The model under review builds one solid part; all positions refer to its coordinate system, in mm. Round coordinates to 2 decimals unless told otherwise and drop trailing zeros. Write each loop counter-clockwise with the first axis right and the second up, starting at its lowest first coordinate (ties: lowest second). Pieces come first, ordered by that corner, then holes. Notation, with made-up numbers: M -4,16.5 L 43,16.5 A25 cw 43,31.5 Z; hole C 27,5 d5. An arc over 180 degrees is marked long. Write item = value, one per line. Start each with the question number.
Item 1: To check wall thickness, follow line 1 along Y through (x, z) = (-27.94, -17.6). State the ranges of the line that lie inside material, in increasing order.
Item 2: The part is to be moulded in two halves that separate along Y. For faces 1 (the cylindrical face through (-28.448, 28.916, -17.866)), 2 (the flat face through (0, 0, -17.25)), say which applies: +Y half, -Y half, draft (parallel to the pull), parting line (faces both ways), or undercut.
Item 3: Take a section at A-A, the plane y = -27.94. Give the boundary of the cut face in (x, z).
Autodesk Inventor part; units mm, degrees
ref_plane "YZ Plane" through (0, 0, 0) normal (1, 0, 0) x (0, 1, 0)
ref_plane "XZ Plane" through (0, 0, 0) normal (0, 1, 0) x (-1, 0, 0)
ref_plane "XY Plane" through (0, 0, 0) normal (0, 0, 1) x (1, 0, 0)
sketch "Skizze1" plane through (0, 0, 0) normal (0, 0, 1) x (1, 0, 0)
  line L0 (-33.02, -33.02) -> (33.02, -33.02)
  line L1 (33.02, -33.02) -> (33.02, 33.02)
  line L2 (33.02, 33.02) -> (-33.02, 33.02)
  line L3 (-33.02, 33.02) -> (-33.02, -33.02)
  line L4 (-33.02, -33.02) -> (33.02, 33.02) construction
  line L5 (33.02, -33.02) -> (-33.02, 33.02) construction
  line L6 (-34, -34) -> (34, -34)
  line L7 (34, -34) -> (34, 34)
  line L8 (34, 34) -> (-34, 34)
  line L9 (-34, 34) -> (-34, -34)
  line L10 (-34, -34) -> (34, 34) construction
  line L11 (34, -34) -> (-34, 34) construction
  point P0 (0, 0)
  dimension "d0" = 66.04
  dimension "d1" = 66.04
  dimension "d2" = 68
  dimension "d3" = 68
extrude "Extrusion1" add sketch "Skizze1" along normal blind 6.5
sketch "Skizze2" plane through (0, 0, 6.5) normal (0, 0, 1) x (1, 0, 0)
  line L0 (-33.02, 33.02) -> (33.02, 33.02)
  line L1 (-33.02, -33.02) -> (33.02, -33.02)
  line L2 (33.02, -33.02) -> (33.02, 33.02)
  line L3 (33.02, 33.02) -> (-33.02, 33.02)
  line L4 (-33.02, 33.02) -> (-33.02, -33.02)
  line L5 (-33.02, -33.02) -> (33.02, 33.02) construction
  line L6 (33.02, -33.02) -> (-33.02, 33.02) construction
  line L7 (34, -34) -> (34, 34)
  line L8 (34, 34) -> (-34, 34)
  line L9 (-34, 34) -> (-34, -34)
  line L10 (-34, -34) -> (34, -34)
  line L11 (-33.02, -33.02) -> (-33.02, 33.02)
  line L12 (-33.02, 33.02) -> (33.02, 33.02)
  line L13 (33.02, 33.02) -> (33.02, -33.02)
  line L14 (33.02, -33.02) -> (-33.02, -33.02)
  point P0 (0, 0)
extrude "Extrusion2" add sketch "Skizze2" along normal blind 2 contours L0 L2 L1 L4 | L10 L9 L8 L7
sketch "Skizze3" plane through (0, 0, 6.5) normal (0, 0, -1) x (-1, 0, 0)
  line L0 (-27.94, -27.94) -> (27.94, -27.94)
  line L1 (27.94, -27.94) -> (27.94, 27.94)
  line L2 (27.94, 27.94) -> (-27.94, 27.94)
  line L3 (-27.94, 27.94) -> (-27.94, -27.94)
  line L4 (-27.94, -27.94) -> (27.94, 27.94) construction
  line L5 (27.94, -27.94) -> (-27.94, 27.94) construction
  circle A0 centre (-27.94, 27.94) radius 3.35
  circle A1 centre (27.94, 27.94) radius 3.35
  circle A2 centre (27.94, -27.94) radius 3.35
  circle A3 centre (-27.94, -27.94) radius 3.35
  point P0 (0, 0)
  dimension "d8" = 55.88
  dimension "d9" = 55.88
  dimension "d10" = 6.7
  dimension "d11" = 6.7
  dimension "d12" = 6.7
  dimension "d13" = 6.7
extrude "Extrusion3" add sketch "Skizze3" along normal blind 5 contours L3 A3 L0 | L0 A3 L3 | A2 L1 L0 | L0 L1 A2 | A0 L2 L3 | L3 L2 A0 | A1 L2 L1 | L1 L2 A1
sketch "Skizze4" plane through (27.94, 27.94, 1.5) normal (0, 0, -1) x (-1, 0, 0)
  circle A0 centre (0, 0) radius 1.1
  circle A1 centre (55.88, 0) radius 3.35
  circle A2 centre (55.88, 0) radius 1.1
  circle A3 centre (55.88, -55.88) radius 3.35
  circle A4 centre (55.88, -55.88) radius 1.1
  circle A5 centre (0, -55.88) radius 3.35
  circle A6 centre (0, -55.88) radius 1.1
  point P0 (27.94, -27.94)
  dimension "d17" = 2.2
  dimension "d18" = 2.2
  dimension "d19" = 2.2
  dimension "d20" = 2.2
extrude "Extrusion4" cut sketch "Skizze4" against normal blind 5 contours A0 | A2 | A4 | A6
sketch "Skizze5" plane through (0, 0, 0) normal (0, 0, -1) x (-1, 0, 0)
  line L0 (-34, -34) -> (-34, 34)
  line L1 (34, -34) -> (-34, -34)
  line L2 (34, 34) -> (34, -34)
  line L3 (-34, 34) -> (34, 34)
  line L4 (33.02, -33.02) -> (33.02, 33.02)
  line L5 (-33.02, -33.02) -> (33.02, -33.02)
  line L6 (-33.02, 33.02) -> (-33.02, -33.02)
  line L7 (33.02, 33.02) -> (-33.02, 33.02)
  point P0 (0, 0)
extrude "Extrusion5" add sketch "Skizze5" along normal blind 4
sketch "Skizze6" plane through (0, 0, -4) normal (0, 0, -1) x (-1, 0, 0)
  line L0 (-33.02, -33.02) -> (33.02, -33.02)
  line L1 (33.02, -33.02) -> (33.02, 33.02)
  line L2 (33.02, 33.02) -> (-33.02, 33.02)
  line L3 (-33.02, 33.02) -> (-33.02, -33.02)
  line L4 (-33.02, -33.02) -> (33.02, 33.02) construction
  line L5 (33.02, -33.02) -> (-33.02, 33.02) construction
  line L6 (33.02, -33.02) -> (20.02, -33.02)
  line L7 (-33.02, -33.02) -> (33.02, -33.02)
  line L8 (20.02, -33.02) -> (10.08, -33.02)
  line L9 (34, -34) -> (-34, -34)
  line L10 (10.08, -33.02) -> (20.02, -33.02)
  line L11 (20.02, -33.02) -> (20.02, -34)
  line L12 (20.02, -34) -> (10.08, -34)
  line L13 (10.08, -34) -> (10.08, -33.02)
  point P0 (0, 0)
  point P1 (-24.13, -33.02)
  point P2 (24.13, -33.02)
  dimension "d25" = 66.04
  dimension "d26" = 66.04
  dimension "d27" = 13
  dimension "d28" = 9.94
extrude "Extrusion6" cut sketch "Skizze6" against normal blind 4 contours L0 L11 L9 L13
fillet "Rundung2" radius 1.75 2 edges at (-10.08, -33.51, 0) (-20.02, -33.51, 0)
sketch "Skizze7" plane through (0, 0, -4) normal (0, 0, -1) x (-1, 0, 0)
  line L0 (34, 34) -> (-34, 34)
  line L1 (-34, -34) -> (34, -34)
  line L2 (34, -34) -> (34, 34)
  line L3 (34, 34) -> (-34, 34)
  line L4 (-34, 34) -> (-34, -34)
  line L5 (-34, -34) -> (34, 34) construction
  line L6 (34, -34) -> (-34, 34) construction
  line L7 (-35, -35) -> (35, -35)
  line L8 (35, -35) -> (35, 35)
  line L9 (35, 35) -> (-35, 35)
  line L10 (-35, 35) -> (-35, -35)
  line L11 (-35, -35) -> (35, 35) construction
  line L12 (35, -35) -> (-35, 35) construction
  point P0 (0, 0)
  point P1 (-34, 34)
  dimension "d32" = 70
  dimension "d33" = 70
extrude "Extrusion7" add sketch "Skizze7" against normal up to surface (12.5 mm away)
sketch "Skizze8" plane through (-20.02, -34, -4) normal (0, 1, 0) x (1, 0, 0)
  line L0 (9.94, -2.25) -> (9.94, 0)
  line L1 (0, 0) -> (9.94, 0)
  line L2 (0, 0) -> (0, -2.25)
  arc A0 (0, -2.25) -> (1.75, -4) centre (1.75, -2.25) ccw
  line L3 (1.75, -4) -> (8.19, -4)
  arc A1 (8.19, -4) -> (9.94, -2.25) centre (8.19, -2.25) ccw
  point P0 (20.02, -4)
extrude "Extrusion8" cut sketch "Skizze8" against normal blind 10
sketch "Skizze9" plane through (0, 0, -4) normal (0, 0, -1) x (-1, 0, 0)
  line L0 (-33.52, 33.52) -> (33.52, 33.52)
  line L1 (33.52, 33.52) -> (33.52, -33.52)
  line L2 (33.52, -33.52) -> (-33.52, -33.52)
  line L3 (-33.52, -33.52) -> (-33.52, 33.52)
  line L4 (-33.52, 33.52) -> (33.52, -33.52) construction
  line L5 (33.52, 33.52) -> (-33.52, -33.52) construction
  line L6 (10.08, -35) -> (10.08, -33.02)
  line L7 (10.08, -33.02) -> (-33.02, -33.02)
  line L8 (-33.02, -33.02) -> (-33.02, 33.02)
  line L9 (-33.02, 33.02) -> (33.02, 33.02)
  line L10 (33.02, 33.02) -> (33.02, -33.02)
  line L11 (33.02, -33.02) -> (20.02, -33.02)
  line L12 (20.02, -33.02) -> (20.02, -35)
  line L13 (20.02, -35) -> (35, -35)
  line L14 (35, -35) -> (35, 35)
  line L15 (35, 35) -> (-35, 35)
  line L16 (-35, 35) -> (-35, -35)
  line L17 (-35, -35) -> (10.08, -35)
  point P0 (0, 0)
  point P1 (10.08, -33.52)
  point P2 (20.02, -33.52)
  dimension "d38" = 67.04
  dimension "d39" = 67.04
extrude "Extrusion9" cut sketch "Skizze9" against normal up to surface (10.5 mm away) contours L0 L1 L2 L12 L11 L10 L9 L8 L7 L6 L3
fillet "Rundung3" radius 2 4 edges at (31.29, -27.94, 6.5) (31.29, 27.94, 6.5) (-24.59, 27.94, 6.5) (-24.59, -27.94, 6.5)
sketch "Skizze10" plane through (-35, -35, -4) normal (-1, 0, 0) x (0, 0, 1)
  point P0 (4, 35)
sketch "Skizze11" plane through (0, 0, 8.5) normal (0, 0, 1) x (1, 0, 0)
  point P0 (0, 0)
sketch "Skizze12" plane through (-18.27, -33.02, 0) normal (0, 1, 0) x (1, 0, 0)
  line L0 (-1.75, 1.75) -> (-1.75, -6.5)
  line L1 (8.19, -6.5) -> (-1.75, -6.5)
  line L2 (8.19, -6.5) -> (8.19, 1.75)
  arc A0 (6.44, 0) -> (8.19, 1.75) centre (6.44, 1.75) ccw
  line L3 (6.44, 0) -> (0, 0)
  arc A1 (-1.75, 1.75) -> (0, 0) centre (0, 1.75) ccw
  point P0 (18.27, 0)
extrude "Extrusion10" cut sketch "Skizze12" against normal up to surface (0.5 mm away)
sketch "Skizze13" plane through (0, 0, -4) normal (0, 0, -1) x (-1, 0, 0)
  circle A0 centre (0, 0) radius 4
  line L0 (0, 0) -> (-10.0581, 1.7135)
  line L1 (0, 0) -> (10.203, 0) construction
  line L2 (0, 0) -> (1.8539, 9.7483)
  line L3 (0, 0) -> (9.923, 0) construction
  line L4 (0, 0) -> (9.888, -2.1637)
  line L5 (0, 0) -> (10.122, 0) construction
  line L6 (0, 0) -> (-2.0234, -10.1982)
  line L7 (0, 0) -> (10.397, 0) construction
  circle A1 centre (-2.0234, -10.1982) radius 2.5
  circle A2 centre (-10.0581, 1.7135) radius 2.5
  circle A3 centre (1.8539, 9.7483) radius 2.5
  circle A4 centre (9.888, -2.1637) radius 2.5
  dimension "d59" = 8
  dimension "d60" = 10.203
  dimension "d61" = 170.332
  dimension "d62" = 9.923
  dimension "d63" = 79.232
  dimension "d64" = 10.122
  dimension "d65" = 12.343
  dimension "d66" = 10.397
  dimension "d67" = 101.222
  dimension "d68" = 5
  dimension "d69" = 5
  dimension "d70" = 5
  dimension "d71" = 5
extrude "Extrusion11" add sketch "Skizze13" against normal up to surface (10.5 mm away) contours A1 | A2 | A3 | A4
sketch "Skizze14" plane through (-9.888, -2.1637, -4) normal (0, 0, -1) x (-1, 0, 0)
  circle A0 centre (0, 0) radius 2.5
  circle A1 centre (-11.9114, -8.0345) radius 2.5
  circle A2 centre (-19.9461, 3.8772) radius 2.5
  circle A3 centre (-8.0341, 11.912) radius 2.5
  point P0 (-9.888, 2.1637)
extrude "Extrusion12" cut sketch "Skizze14" against normal blind 5.5
fillet "Rundung4" radius 4 4 edges at (12.5581, 1.7135, 6.5) (0.6461, 9.7483, 6.5) (-7.388, -2.1637, 6.5) (4.5234, -10.1982, 6.5)
sketch "Skizze15" plane through (-9.888, -2.1637, 1.5) normal (0, 0, -1) x (-1, 0, 0)
  circle A0 centre (0, 0) radius 1
  circle A1 centre (-11.9114, -8.0345) radius 2.5
  circle A2 centre (-11.9114, -8.0345) radius 1
  circle A3 centre (-19.9461, 3.8772) radius 2.5
  circle A4 centre (-19.9461, 3.8772) radius 1
  circle A5 centre (-8.0341, 11.912) radius 2.5
  circle A6 centre (-8.0341, 11.912) radius 1
  point P0 (-9.888, 2.1637)
  dimension "d77" = 2
  dimension "d78" = 2
  dimension "d79" = 2
  dimension "d80" = 2
extrude "Extrusion13" cut sketch "Skizze15" against normal blind 5 contours A0 | A2 | A4 | A6
chamfer "Fase1" distance 4 angle 45 4 edges at (-33.52, 0, 6.5) (0, -33.52, 6.5) (0, 33.52, 6.5) (33.52, 0, 6.5)
sketch "Skizze16" plane through (10.0581, 1.7135, 1.5) normal (0, 0, -1) x (-1, 0, 0)
  circle A0 centre (0, 0) radius 1.6
  circle A1 centre (8.0347, -11.9117) radius 1
  circle A2 centre (8.0347, -11.9117) radius 1.6
  circle A3 centre (11.912, 8.0348) radius 1
  circle A4 centre (11.912, 8.0348) radius 1.6
  circle A5 centre (19.9461, -3.8772) radius 1
  circle A6 centre (19.9461, -3.8772) radius 1.6
  point P0 (10.0581, -1.7135)
  dimension "d86" = 3.2
  dimension "d87" = 3.2
  dimension "d88" = 3.2
  dimension "d89" = 3.2
extrude "Extrusion14" cut sketch "Skizze16" against normal blind 10 contours A0 | A1 | A2 | A3 | A4 | A5 | A6
chamfer "Fase2" distance 2 angle 45 4 edges at (-8.288, -2.1637, 8.5) (3.6234, -10.1982, 8.5) (11.6581, 1.7135, 8.5) (-0.2539, 9.7483, 8.5)
sketch "Skizze17" plane through (27.94, 27.94, 1.5) normal (0, 0, -1) x (-1, 0, 0)
  circle A0 centre (0, 0) radius 1.1
  circle A1 centre (0, 0) radius 3.35
  circle A2 centre (55.88, 0) radius 1.1
  circle A3 centre (55.88, 0) radius 3.35
  circle A4 centre (55.88, -55.88) radius 1.1
  circle A5 centre (55.88, -55.88) radius 3.35
  circle A6 centre (0, -55.88) radius 1.1
  circle A7 centre (0, -55.88) radius 3.35
  line L0 (61.46, 5.58) -> (58.4446, 2.5646)
  line L1 (-2.5646, -58.4446) -> (58.4446, -58.4446)
  line L2 (58.4446, -58.4446) -> (58.4446, 2.5646)
  line L3 (58.4446, 2.5646) -> (-2.5646, 2.5646)
  line L4 (-2.5646, 2.5646) -> (-2.5646, -58.4446)
  line L5 (-2.5646, -58.4446) -> (58.4446, 2.5646) construction
  line L6 (58.4446, -58.4446) -> (-2.5646, 2.5646) construction
  point P0 (27.94, -27.94)
extrude "Extrusion15" add sketch "Skizze17" along normal blind 20 contours A1 L4 L3 | A1 L3 A3 L2 A5 L1 A7 L4 | A1 L4 L3 | L3 A3 L2 | A7 L1 L4 | L3 L2 A3 | A7 L1 L4 | L2 A5 L1 | L2 L1 A5
sketch "Skizze18" plane through (0, 0, 8.5) normal (0, 0, 1) x (1, 0, 0)
  line L0 (-192.7529, 161.1187) -> (54.5088, 161.1187)
  line L1 (54.5088, 161.1187) -> (54.5088, -50.2743)
  line L2 (54.5088, -50.2743) -> (-192.7529, -50.2743)
  line L3 (-192.7529, -50.2743) -> (-192.7529, 161.1187)
  line L4 (-192.7529, 161.1187) -> (54.5088, -50.2743) construction
  line L5 (54.5088, 161.1187) -> (-192.7529, -50.2743) construction
  point P0 (0, 0)
  point P1 (-69.122, 55.4222)
extrude "Extrusion16" cut sketch "Skizze18" against normal blind 25.75
properties part number "bottomplate_3D-Druck"
Response values:
q1.line_1 = -30.5 to -29.04, -26.84 to 26.84, 29.04 to 30.5
q2.face_1 = undercut
q2.face_2 = draft
q3.outline = M -30.5,-18.5 L -29.04,-18.5 L -29.04,-17.25 L -30.5,-17.25 Z; M -26.84,-18.5 L 26.84,-18.5 L 26.84,-17.25 L -26.84,-17.25 Z; M 29.04,-18.5 L 30.5,-18.5 L 30.5,-17.25 L 29.04,-17.25 Z
